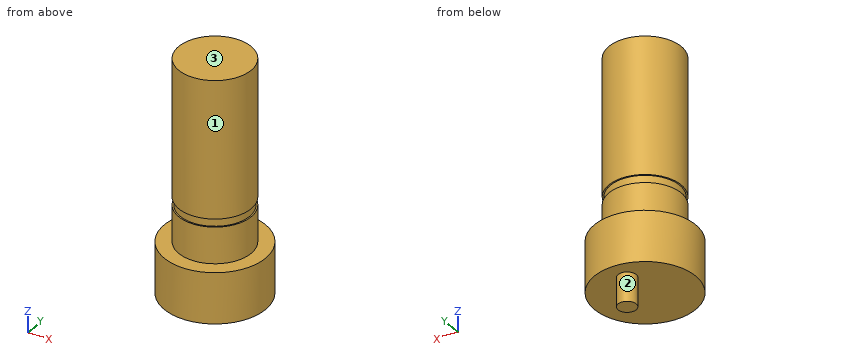
from build123d import *

# Parameters (mm, degrees)
SKETCH1_R           = 7
BOSS_EXTRUDE1_DEPTH = 7
SKETCH2_R           = 5
BOSS_EXTRUDE2_DEPTH = 25
SKETCH3_R           = 6
SKETCH3_R_2         = 4.8
CUT_EXTRUDE1_DEPTH  = 1.1
SKETCH4_R           = 1.25
BOSS_EXTRUDE3_DEPTH = 4


with BuildPart() as part:
    # Sketch1 → Boss-Extrude1 (new body)
    with BuildSketch(Plane.XY):
        Circle(SKETCH1_R)
    extrude(amount=-BOSS_EXTRUDE1_DEPTH)

    # Sketch2 → Boss-Extrude2 (add)
    with BuildSketch(Plane.XY):
        Circle(SKETCH2_R)
    extrude(amount=BOSS_EXTRUDE2_DEPTH)

    # Sketch3 → Cut-Extrude1 (cut)
    with BuildSketch(Plane.XY.offset(5)):
        Circle(SKETCH3_R)
        Circle(SKETCH3_R_2, mode=Mode.SUBTRACT)
    extrude(amount=CUT_EXTRUDE1_DEPTH, mode=Mode.SUBTRACT)

    # Sketch4 → Boss-Extrude3 (add)
    with BuildSketch(Plane(origin=(0, 0, -7), x_dir=(-1, 0, 0), z_dir=(0, 0, -1))):
        with Locations((0, 4)):
            Circle(SKETCH4_R)
    extrude(amount=BOSS_EXTRUDE3_DEPTH)


solid = part.part
CAD build for the part. Positions are in the model's coordinates, mm. Face numbers are marked on the shaded views. A direction names the side the tool comes from. Round coordinates to 2 decimals unless told otherwise and drop trailing zeros. Loops run counter-clockwise (first coordinate to the right, second up) from the corner with the lowest first, then second, coordinate; pieces in that order, holes last.
(1) Cut at A-A (x = 0). Give the cut face in (y, z), plus the area to 3 significant figures.
(2) Cut at B-B (y = 3.25). Give the cut face in (x, z), plus the area to 3 significant figures.
(3) Which spindle directions (+Z, -Z, +X, -X, +Y, -Y) get a long thin tool onto all of the face, cutting with end or side? Do the marked faces 1, 2 and 3. Say none if no direction does.
(4) Wall check: line 1 along Z through (x, y) = (-3.5, -4.25); line 2 along Z through (x, y) = (0.5, -0.5); line 3 along X through (y, z) = (0.25, 2). Give the ranges that are in metal, low to high.
(5) Cut at D-D (x = 3.25). Give the cut face in (y, z), plus the area to 3 significant figures.
(6) Cut at C-C (z = 13.5). Give the cut face in (x, y).
(7) Drop flat-ended pins along their axis: pin 1 (4 mm diameter, centred on y = -1, z = 14.5, fed in from -X); pin 2 (1.5 mm diameter, centred on y = 0, z = 1, fed in from +X); pin 3 (8 mm diameter, centred on y = 2.5, z = -4, fed in from +X); pin 4 (5 mm diameter, centred on y = -5.5, z = 17.5, fed in from -X). Give the stop position or say it passes through.
Findings below:
1. outline: (-7, -7) - (2.75, -7) - (2.75, -11) - (5.25, -11) - (5.25, -7) - (7, -7) - (7, 0) - (5, 0) - (5, 5) - (4.8, 5) - (4.8, 6.1) - (5, 6.1) - (5, 25) - (-5, 25) - (-5, 6.1) - (-4.8, 6.1) - (-4.8, 5) - (-5, 5) - (-5, 0) - (-7, 0) - close
1. area: 358 mm2
2. outline: (-6.2, -7) - (-1, -7) - (-1, -11) - (1, -11) - (1, -7) - (6.2, -7) - (6.2, 0) - (3.8, 0) - (3.8, 5) - (3.53, 5) - (3.53, 6.1) - (3.8, 6.1) - (3.8, 25) - (-3.8, 25) - (-3.8, 6.1) - (-3.53, 6.1) - (-3.53, 5) - (-3.8, 5) - (-3.8, 0) - (-6.2, 0) - close
2. area: 284 mm2
3. face 1: +Z
3. face 2: -Z
3. face 3: +Z, +X, -X, +Y, -Y
4. line 1: z = -7 to 0
4. line 2: z = -7 to 25
4. line 3: x = -4.99 to 4.99
5. outline: (-6.2, -7) - (6.2, -7) - (6.2, 0) - (3.8, 0) - (3.8, 5) - (3.53, 5) - (3.53, 6.1) - (3.8, 6.1) - (3.8, 25) - (-3.8, 25) - (-3.8, 6.1) - (-3.53, 6.1) - (-3.53, 5) - (-3.8, 5) - (-3.8, 0) - (-6.2, 0) - close
5. area: 276 mm2
6. outline: circle Ø10 at (0, 0)
7. pin 1: stops at x = -5
7. pin 2: stops at x = 5
7. pin 3: stops at x = 7
7. pin 4: stops at x = -4
